Input: part model. Units: mm. Frame: model coordinates. A direction names the side the tool comes from. Give positions to 0.01 mm unless a question says otherwise; leave off trailing zeros. Write each loop counter-clockwise with the first axis right and the second up, starting at its lowest first coordinate (ties: lowest second). Pieces come first, ordered by that corner, then holes. Notation, with made-up numbers: (80.5, -28) -> (87.5, -28) arc R27 ccw to (87.5, 9) -> close; hole circle Ø1 at (89.25, -5). An arc over 180 degrees is marked (long way). Return JSON: item names as keys, results as strings. Group by question number.
Item 1: Section B-B, the plane z = 15. Return loops of the section in (x, y), then the cut area to 3 significant figures.
Item 2: Mould query, pull axis Y, two halves, no side actions, for faces 3 (the face through (0, 20, 15)), 4 (the face through (0, -17, 0)), 5 (the face through (23.365, -10.2, 14.8)). Classes: released by +Y, released by -Y, zero draft, split by the parting line, or undercut.
Item 3: Section A-A, the plane y = 0. Return loops of the section in (x, z), then the cut area to 3 significant figures.
Item 4: Section C-C, the plane x = 14.5. Return loops of the section in (y, z).
Item 5: Line query: line 1 (Y direction, x = 27.1, z = 15); line 2 (Y direction, x = -6.5, z = 22.75); line 3 (X direction, y = -7, z = 6.75). Output: solid intervals per line, ascending. Write a range as [from, to].
Item 6: Set-up query: faces 1 (the face through (0, -15, 15)), 2 (the face through (0, -20, 15)). Return all of +Z, -Z, +X, -X, +Y, -Y with unobstructed straight access to the full face (end or side cutting, diameter ignored); none if empty.
Item 7: Section D-D, the plane x = -24. Return loops of the section in (y, z).
from build123d import *

# Parameters (mm, degrees)
SKETCH1_W           = 56.729559748
SKETCH1_H           = 40
SKETCH1_W_2         = 46.729559748
SKETCH1_H_2         = 30
EXTRUDE_THIN1_DEPTH = 30
SKETCH2_R           = 10
CUT_EXTRUDE1_DEPTH  = 68.217876709


with BuildPart() as part:
    # Sketch1 → Extrude-Thin1 (new body)
    with BuildSketch(Plane.XY):
        Rectangle(SKETCH1_W, SKETCH1_H)
        Rectangle(SKETCH1_W_2, SKETCH1_H_2, mode=Mode.SUBTRACT)
    extrude(amount=EXTRUDE_THIN1_DEPTH)

    # Sketch2 → Cut-Extrude1 (cut, through all)
    with BuildSketch(Plane.ZY.offset(28.364779874)):
        with Locations((15, 0)):
            Circle(SKETCH2_R)
    extrude(amount=-CUT_EXTRUDE1_DEPTH, mode=Mode.SUBTRACT)


solid = part.part
Answer below:
{
 "1": {"outline": "(-28.36, -20) -> (28.36, -20) -> (28.36, -10) -> (23.36, -10) -> (23.36, -15) -> (-23.36, -15) -> (-23.36, -10) -> (-28.36, -10) -> close; (-28.36, 10) -> (-23.36, 10) -> (-23.36, 15) -> (23.36, 15) -> (23.36, 10) -> (28.36, 10) -> (28.36, 20) -> (-28.36, 20) -> close", "area": "667 mm2"},
 "2": {"face 3": "released by +Y", "face 4": "zero draft", "face 5": "undercut"},
 "3": {"outline": "(-28.36, 0) -> (-23.36, 0) -> (-23.36, 5) -> (-28.36, 5) -> close; (-28.36, 25) -> (-23.36, 25) -> (-23.36, 30) -> (-28.36, 30) -> close; (23.36, 0) -> (28.36, 0) -> (28.36, 5) -> (23.36, 5) -> close; (23.36, 25) -> (28.36, 25) -> (28.36, 30) -> (23.36, 30) -> close", "area": "100 mm2"},
 "4": {"outline": "(-20, 0) -> (-15, 0) -> (-15, 30) -> (-20, 30) -> close; (15, 0) -> (20, 0) -> (20, 30) -> (15, 30) -> close"},
 "5": {"line 1": "y = [-20, -10], [10, 20]", "line 2": "y = [-20, -15], [15, 20]", "line 3": "x = [-28.36, -23.36], [23.36, 28.36]"},
 "6": {"face 1": "+Z, -Z", "face 2": "+Z, -Z, +X, -X, -Y"},
 "7": {"outline": "(-20, 0) -> (20, 0) -> (20, 30) -> (-20, 30) -> close; hole circle Ø20 at (0, 15)"}
}
